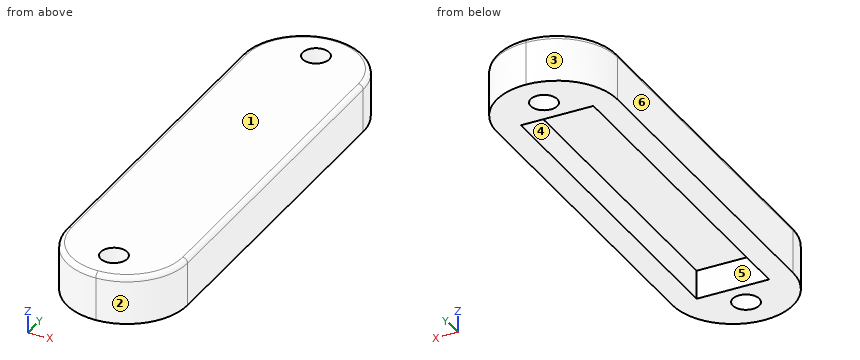
```python
from build123d import *

# Parameters (mm, degrees)
F0_W     = 25
F0_H     = 95
F0_R     = 2.75
F1_DEPTH = 10
F2_R     = 12.49999
F3_R     = 1
F4_W     = 15
F4_H     = 70
F5_DEPTH = 6


# Not quite as in the source:
# - a fillet or chamfer is up to 0.001 mm smaller than in the source, because OpenCascade refuses the exact size


with BuildPart() as f1:
    # F0 (on Top) → F1 (new body)
    with BuildSketch(Plane.XY):
        with Locations((12.5, 47.5)):
            Rectangle(F0_W, F0_H)
        with Locations((12.5, 7.25)):
            Circle(F0_R, mode=Mode.SUBTRACT)
        with Locations((12.5, 87.75)):
            Circle(F0_R, mode=Mode.SUBTRACT)
    extrude(amount=F1_DEPTH)

    # F2 (radius 12.5 in the source; OpenCascade refuses exactly that, so slightly less here)
    f2_edges = [f1.edges().sort_by_distance(p)[0] for p in [
        (25, 95, 5),
        (0, 95, 5),
        (25, 0, 5),
        (0, 0, 5),
    ]]
    fillet(f2_edges, radius=F2_R)

    # F3
    f3_edges = [f1.edges().sort_by_distance(p)[0] for p in [
        (25, 47.5, 10),
        (0, 47.5, 10),
        (12.5, 95, 10),
        (21.338838, 91.338838, 10),
        (3.661162, 91.338838, 10),
        (21.338838, 3.661162, 10),
        (12.5, 0, 10),
        (3.661162, 3.661162, 10),
    ]]
    fillet(f3_edges, radius=F3_R)

    # F4 (on face) → F5 (cut)
    with BuildSketch(Plane(origin=(0, 0, 0), x_dir=(1, 0, 0), z_dir=(0, 0, -1))):
        with Locations((12.5, -47.5)):
            Rectangle(F4_W, F4_H)
    extrude(amount=-F5_DEPTH, mode=Mode.SUBTRACT)


solid = f1.part
```
Can you work these out from the model? Positions are in its coordinate system, mm. Face numbers are marked on the shaded views. A direction names the side the tool comes from. Coordinates: 2 decimals unless noted, no trailing zeros. Loops run counter-clockwise (first coordinate to the right, second up) from the corner with the lowest first, then second, coordinate; pieces in that order, holes last. Notation, with made-up numbers: (-11.75, -5) - (22.25, -5) arc R23 ccw to (22.25, 31) - close; hole circle Ø1 at (-36, 61.5). An arc over 180 degrees is marked (long way). Use a Markdown table: item, result.
Item 1: We'd pull the mould along Y, two halves only. Please class the marked faces 1, 2, 3 and 4: released by +Y, released by -Y, zero draft, split by the parting line, or undercut.
Numbers:
| item | result |
|---|---|
| face 1 | zero draft |
| face 2 | released by -Y |
| face 3 | released by +Y |
| face 4 | undercut |
Item 2: I want a section at C-C on y = 45.5. Please give me the cut outline in (x, z).
Numbers:
| item | result |
|---|---|
| outline | (0, 0) - (5, 0) - (5, 6) - (20, 6) - (20, 0) - (25, 0) - (25, 9) arc R1 ccw to (24, 10) - (1, 10) arc R1 ccw to (0, 9) - close |
Item 3: For the marked faces 5 and 6, which set-ups out of +Z, -Z, +X, -X, +Y, -Y let a thin tool reach every point of the face, with its end or its side?
Numbers:
| item | result |
|---|---|
| face 5 | -Z |
| face 6 | +Z, -Z, -X, +Y, -Y |
Item 4: If I drill on probe 1 along Y at (x, z) = (12.5, 3); probe 2 along Y at (x, z) = (12.5, 6.75); probe 3 along Y at (x, z) = (11.75, 1), over which ranges is the centre line in solid material (lowest first)? Write a range as from..to.
Numbers:
| item | result |
|---|---|
| probe 1 | y = 0..4.5, 10..12.5, 82.5..85, 90.5..95 |
| probe 2 | y = 0..4.5, 10..85, 90.5..95 |
| probe 3 | y = 0.02..4.6, 9.9..12.5, 82.5..85.1, 90.4..94.98 |
Item 5: I want a section at A-A on z = 7.5. Give the number of separate pieces and of enclosed holes in the cut face, and give its area (3 significant figures).
Numbers:
| item | result |
|---|---|
| separate pieces | 1 |
| enclosed holes | 2 |
| area | 2,190 mm2 |
Item 6: Will these pins go through, and if not, where does the flat tip stop? pin 1 (2 mm diameter, centred on x = 21, z = 6.5, fed in from -Y); pin 2 (4 mm diameter, centred on x = 3, z = 5.5, fed in from +Y); pin 3 (4.5 mm diameter, centred on x = 10, y = 65, fed in from -Z).
Numbers:
| item | result |
|---|---|
| pin 1 | stops at y = 2.5 |
| pin 2 | stops at y = 92.5 |
| pin 3 | stops at z = 6 |
